The model under review builds one solid part; all positions refer to its coordinate system, in mm. A direction names the side the tool comes from. Coordinates: 2 decimals unless noted, no trailing zeros. Order: outer loops, then holes, each group sorted by start corner. A loop starts at its lowest first (then second) coordinate and runs counter-clockwise, first axis right, second up.
```python
from build123d import *

# Parameters (mm, degrees)
F1_DEPTH = 80.625
F2_T     = -2.54


# Not quite as in the source:
# - a shell that OpenCascade refuses in one call is made with other operations: the cavity is built on its own and cut out


with BuildPart() as f1:
    # F0 (on Front) → F1 (new body)
    with BuildSketch(Plane.XZ):
        Polygon((0, 7.1409749798), (0, 0), (56.7328892648, 0), (56.7328892648, 71.0757300258), (50.1917116344, 71.0757300258), (50.1917116344, 7.1409749798), align=None)
    extrude(amount=F1_DEPTH)

    # F2: a shell. OpenCascade refuses it in one call, so the cavity is built on its own and cut out:
    # the body offset inwards by the wall thickness, plus a prism from it out through each open face.
    f2_core = offset(f1.part, amount=F2_T, kind=Kind.INTERSECTION, mode=Mode.PRIVATE)
    f2_exits = [f2_core.faces().sort_by_distance(p)[0] for p in [
        (52.731712, -40.3125, 36.568353),
    ]]
    add(f2_core, mode=Mode.SUBTRACT)
    extrude(f2_exits, amount=-F2_T, mode=Mode.SUBTRACT)


solid = f1.part
```
(1) Draft analysis for pull direction X (two halves, no side actions). For faces 1 (the face through (52, -40, 68.536)), 2 (the face through (0, -40, 4)), 3 (the face through (28, -40, 2.54)), state which applies: released by +X, released by -X, zero draft, split by the parting line, or undercut.
A:
face 1: zero draft
face 2: released by -X
face 3: undercut
(2) For pin 1 Ø1.5 at (x, y) = (45, -28) entering from +Z; pin 2 Ø8 at (x, z) = (21.5, 12.5) entering from +Y, all flat-tipped, find the tip position at first contact; note any pin that passes through.
A:
pin 1: stops at z = 7.14
pin 2: passes through
(3) Machinability: for faces 4 (the face through (50.192, -40, 70)), 5 (the face through (50.192, -40, 6)), 6 (the face through (54, -40, 71.076)), which of the approach directions +Z, -Z, +X, -X, +Y, -Y give a long, thin tool a straight path to every point of the face, cutting with its end or side? Answer none if there is none.
A:
face 4: +Z, -X, +Y, -Y
face 5: none
face 6: +Z, +X, -X, +Y, -Y
(4) We need section C-C, the plane z = 32. Write out the cut boundary in (x, y) (3 decimals), and give its area (3 significant figures).
A:
outline: (50.192, -80.625) - (56.733, -80.625) - (56.733, 0) - (50.192, 0) - (50.192, -2.54) - (54.193, -2.54) - (54.193, -78.085) - (50.192, -78.085) - close
area: 225 mm2
(5) We need section B-B, the plane y = -66. Write out the cut boundary in (x, z).
A:
outline: (0, 0) - (56.73, 0) - (56.73, 71.08) - (50.19, 71.08) - (50.19, 68.54) - (54.19, 68.54) - (54.19, 2.54) - (2.54, 2.54) - (2.54, 4.6) - (50.19, 4.6) - (50.19, 7.14) - (0, 7.14) - close
(6) We need section D-D, the plane x = 52. Write out the cut boundary in (y, z) (3 decimals).
A:
outline: (-80.625, 0) - (0, 0) - (0, 71.076) - (-80.625, 71.076) - close; hole (-78.085, 2.54) - (-2.54, 2.54) - (-2.54, 68.536) - (-78.085, 68.536) - close
(7) Wall thickness on probe 1 along Z at (x, y) = (10, -29); probe 2 along Y at (x, z) = (52, 31.5) (3 decimals); probe 3 along X at (y, z) = (-39.5, 59): over which ranges is each line inside the solid? List them lowest first.
A:
probe 1: z = 0 to 2.54, 4.6 to 7.14
probe 2: y = -80.625 to -78.085, -2.54 to 0
probe 3: x = 54.19 to 56.73
(8) We need section A-A, the plane x = 10. Write out the cut boundary in (y, z) (3 decimals), and give its area (3 significant figures).
A:
outline: (-80.625, 0) - (0, 0) - (0, 7.141) - (-80.625, 7.141) - close; hole (-78.085, 2.54) - (-2.54, 2.54) - (-2.54, 4.601) - (-78.085, 4.601) - close
area: 420 mm2
